Input: part model. Units: mm. Frame: model coordinates. A direction names the side the tool comes from. Round coordinates to 2 decimals unless told otherwise and drop trailing zeros. Loops run counter-clockwise (first coordinate to the right, second up) from the corner with the lowest first, then second, coordinate; pieces in that order, holes last.
1) Section A-A, the plane x = 4.35. Return loops of the section in (y, z), and give its area (3 significant figures).
2) Access query for faces 1 (the face through (47.635, 0.396, -14.142)), 2 (the face through (0, 4, 1)). Directions: +Z, -Z, +X, -X, +Y, -Y. A direction counts if a zero-diameter tool reaches every point of the face in a straight line with its end or side. Return the directions, or none.
3) Section B-B, the plane z = -30. Return loops of the section in (x, y), and give its area (3 significant figures).
4) Section C-C, the plane y = 4.5. Return loops of the section in (x, z), and give its area (3 significant figures).
5) Draft query along Z for faces 3 (the face through (21, 2, -40)), 4 (the face through (48.28, 0.21, -29.5)), 5 (the face through (6, 3, 1)), 6 (the face through (47.635, 0.396, 2.058)). Return one class per face: pulls with the +Z half, pulls with the -Z half, needs draft (parallel to the pull), parting line crosses it, or undercut.
6) Ray query, line 1 along Z through (x, y) = (4.35, 4.5); line 2 along Y through (x, z) = (5, -27); line 3 along Y through (x, z) = (37.5, -27.5) (3 decimals). Return the intervals inside material, ascending.
7) Section D-D, the plane x = 19. Return loops of the section in (y, z).
8) First-contact query: pin 1 (3.5 mm diameter, centred on x = 4.35, z = 30, fed in from -Y); pin 2 (0.9 mm diameter, centred on y = 2, z = -5.5, fed in from -X). Flat tips, straight axial feed; report the tip coordinate or a pass-through.
from build123d import *

# Parameters (mm, degrees)
BOSS_EXTRUDE1_DEPTH = 40
CUT_EXTRUDE1_DEPTH  = 40
SKETCH4_R           = 1.45
CUT_EXTRUDE2_DEPTH  = 40
CHAMFER1_SIZE       = 0.5


with BuildPart() as part:
    # Sketch1 → Boss-Extrude1 (new, symmetric)
    with BuildSketch(Plane.XY):
        Polygon((0, 6), (12, 6), (52, 0), (12, 0), (12, 3), (0, 3), align=None)
    extrude(amount=BOSS_EXTRUDE1_DEPTH, both=True)

    # Sketch3 → Cut-Extrude1 (cut, symmetric)
    with BuildSketch(Plane(origin=(1.144254279, 7.628361858, 0), x_dir=(0.9889363528682976, -0.14834045293024462, 0), z_dir=(0.14834045293024462, 0.9889363528682976, 0))):
        Polygon((51.424690349, -40), (45.424690349, -32.4), (51.424690349, -24.8), align=None)
        Polygon((51.424690349, -23.8), (51.424690349, -8.6), (45.424690349, -16.2), align=None)
        Polygon((51.424690349, -7.6), (51.424690349, 7.6), (45.424690349, 0), align=None)
        Polygon((51.424690349, 8.6), (51.424690349, 23.8), (45.424690349, 16.2), align=None)
        Polygon((51.424690349, 24.8), (51.424690349, 40), (45.424690349, 32.4), align=None)
    extrude(amount=CUT_EXTRUDE1_DEPTH, both=True, mode=Mode.SUBTRACT)

    # Sketch4 → Cut-Extrude2 (cut, symmetric)
    with BuildSketch(Plane(origin=(0, 6, 0), x_dir=(1, 0, 0), z_dir=(0, 1, 0))):
        with Locations(Location((4.35, -30, 0), (0, 0, 180))):
            Circle(SKETCH4_R)
        with Locations(Location((4.35, 30, 0), (0, 0, 180))):
            Circle(SKETCH4_R)
    extrude(amount=CUT_EXTRUDE2_DEPTH, both=True, mode=Mode.SUBTRACT)

    # Chamfer1
    chamfer1_edges = [part.edges().sort_by_distance(p)[0] for p in [
        (5.8, 6, 30),
        (5.8, 6, -30),
    ]]
    chamfer(chamfer1_edges, length=CHAMFER1_SIZE)


solid = part.part
Final values:
1. outline: (3, -40) - (6, -40) - (6, -31.95) - (5.5, -31.45) - (3, -31.45) - close; (3, -28.55) - (5.5, -28.55) - (6, -28.05) - (6, 28.05) - (5.5, 28.55) - (3, 28.55) - close; (3, 31.45) - (5.5, 31.45) - (6, 31.95) - (6, 40) - (3, 40) - close
1. area: 222 mm2
2. face 1: +X, -Y
2. face 2: +Z, -Z, -X, +Y, -Y
3. outline: (0, 3) - (2.9, 3) - (2.9, 5.5) - (2.4, 6) - (0, 6) - close; (5.8, 3) - (12, 3) - (12, 0) - (47.85, 0) - (47.94, 0.61) - (12, 6) - (6.3, 6) - (5.8, 5.5) - close
3. area: 146 mm2
4. outline: (0, -40) - (22, -40) - (22, 40) - (0, 40) - close; hole circle Ø2.9 at (4.35, -30); hole circle Ø2.9 at (4.35, 30)
4. area: 1,750 mm2
5. face 3: pulls with the -Z half
5. face 4: undercut
5. face 5: needs draft
5. face 6: undercut
6. line 1: z = -40 to -31.45, -28.55 to 28.55, 31.45 to 40
6. line 2: y = 3 to 6
6. line 3: y = 0 to 2.175
7. outline: (0, -40) - (4.95, -40) - (4.95, 40) - (0, 40) - close
8. pin 1: stops at y = 3
8. pin 2: stops at x = 12
